from build123d import *

# Parameters (mm, degrees)
F1_DEPTH = 48
F2_R     = 11
F3_DEPTH = 2
F4_R     = 2.5
F5_DEPTH = 24
F6_R     = 1.5
F7_DEPTH = 4


with BuildPart() as f1:
    # F0 (on Top) → F1 (new body)
    with BuildSketch(Plane.XY):
        with BuildLine():
            ThreePointArc((21.15, 14.078932), (17.965785, 17.965785), (14.078932, 21.15))
            Line((14.078932, 21.15), (-14.078932, 21.15))
            ThreePointArc((-14.078932, 21.15), (-17.965785, 17.965785), (-21.15, 14.078932))
            Line((-21.15, 14.078932), (-21.15, -14.078932))
            ThreePointArc((-21.15, -14.078932), (-17.965785, -17.965785), (-14.078932, -21.15))
            Line((-14.078932, -21.15), (14.078932, -21.15))
            ThreePointArc((14.078932, -21.15), (17.965785, -17.965785), (21.15, -14.078932))
            Line((21.15, -14.078932), (21.15, 14.078932))
        make_face()
    extrude(amount=F1_DEPTH)

    # F2 (on face) → F3 (join)
    with BuildSketch(Plane.XY.offset(48)):
        Circle(F2_R)
    extrude(amount=F3_DEPTH)

    # F4 (on face) → F5 (join)
    with BuildSketch(Plane.XY.offset(50)):
        Circle(F4_R)
    extrude(amount=F5_DEPTH)

    # F6 (on face) → F7 (cut)
    with BuildSketch(Plane.XY.offset(48)):
        with Locations((-15.5, -15.5)):
            Circle(F6_R)
        with Locations((15.5, -15.5)):
            Circle(F6_R)
        with Locations((15.5, 15.5)):
            Circle(F6_R)
        with Locations((-15.5, 15.5)):
            Circle(F6_R)
    extrude(amount=-F7_DEPTH, mode=Mode.SUBTRACT)


solid = f1.part
The listing builds one solid part. Answer for the finished solid, in the listing's coordinates (mm). A direction names the side the tool comes from. Coordinates: 2 decimals unless noted, no trailing zeros. Order: outer loops, then holes, each group sorted by start corner. A loop starts at its lowest first (then second) coordinate and runs counter-clockwise, first axis right, second up. Notation, with made-up numbers: (0.25, -25) -> (14.25, -25) arc R27 cw to (14.25, -6) -> close; hole circle Ø4 at (46.5, 44). An arc over 180 degrees is marked (long way). Answer in a Markdown table with one row per item. Add a question column.
Item 1: Find section A-A (x = 0). Write down the section's boundary in (y, z).
Item 2: Each of these flat-tipped pins is pushed along its axis until it touches: P1, Ø10, axis at y = 9, z = 54.5, coming from the +X side; P2, Ø5, axis at x = -3, z = 58.5, coming from the -Y side; P3, Ø4, axis at x = 15.5, y = 15.5, coming from the +Z side; P4, Ø2.5, axis at x = 15.5, y = -15.5, coming from the -Z side. Where does it stop, or does it pass through?
Item 3: Determine the mould class of faces 3 (the face through (0, 0, 0)), 4 (the face through (-17, -15.43, 46.03)), 5 (the face through (17.916, -18.016, 23.664)) for opening direction X: +X half, -X half, draft (parallel to the pull), parting line (faces both ways), or undercut.
Item 4: Which of the six approach directions +Z, -Z, +X, -X, +Y, -Y give full straight-line access (tool end or side, diameter ignored) to faces 1 (the face through (-18.016, -17.916, 23.664)), 2 (the face through (15, -15, 44))?
Item 5: Find section B-B (z = 17). Write down the section's boundary in (x, y), then the cut area to 3 significant figures.
Item 6: Find the intervals of material crossed by L1, parallel to X at y = -15, z = 46; L2, parallel to Z at x = -8.5, y = -11.5, in increasing order. Write a range as from..to.
Item 7: Find section D-D (x = -8). Write down the section's boundary in (y, z).
Result set:
| question | item | result |
|---|---|---|
| 1 | outline | (-21.15, 0) -> (21.15, 0) -> (21.15, 48) -> (11, 48) -> (11, 50) -> (2.5, 50) -> (2.5, 74) -> (-2.5, 74) -> (-2.5, 50) -> (-11, 50) -> (-11, 48) -> (-21.15, 48) -> close |
| 2 | P1 | stops at x = 8.63 |
| 2 | P2 | stops at y = -2.45 |
| 2 | P3 | stops at z = 48 |
| 2 | P4 | stops at z = 0 |
| 3 | face 3 | draft |
| 3 | face 4 | undercut |
| 3 | face 5 | +X half |
| 4 | face 1 | +Z, -Z, -X, -Y |
| 4 | face 2 | +Z |
| 5 | outline | (-21.15, -14.08) arc R25.41 ccw to (-14.08, -21.15) -> (14.08, -21.15) arc R25.41 ccw to (21.15, -14.08) -> (21.15, 14.08) arc R25.41 ccw to (14.08, 21.15) -> (-14.08, 21.15) arc R25.41 ccw to (-21.15, 14.08) -> close |
| 5 | area | 1,700 mm² |
| 6 | L1 | x = -20.51..-16.91, -14.09..14.09, 16.91..20.51 |
| 6 | L2 | z = 0..48 |
| 7 | outline | (-21.15, 0) -> (21.15, 0) -> (21.15, 48) -> (7.55, 48) -> (7.55, 50) -> (-7.55, 50) -> (-7.55, 48) -> (-21.15, 48) -> close |
